from build123d import *

# Parameters (mm, degrees)
F0_W     = 60
F0_H     = 60
F0_R     = 2.2
F0_R_2   = 29
F1_DEPTH = 25
F3_DEPTH = 3


with BuildPart() as f1:
    # F0 (on Top) → F1 (new body)
    with BuildSketch(Plane.XY):
        Rectangle(F0_W, F0_H)
        with Locations((-25, -25)):
            Circle(F0_R, mode=Mode.SUBTRACT)
        with Locations((25, -25)):
            Circle(F0_R, mode=Mode.SUBTRACT)
        with Locations((-25, 25)):
            Circle(F0_R, mode=Mode.SUBTRACT)
        Circle(F0_R_2, mode=Mode.SUBTRACT)
        with Locations((25, 25)):
            Circle(F0_R, mode=Mode.SUBTRACT)
    extrude(amount=F1_DEPTH)

    # F2 (on face) → F3 (join)
    with BuildSketch(Plane.XY.offset(25)):
        with BuildLine():
            Line((-10, 27.221315), (-10, 0))
            ThreePointArc((-10, 0), (-9.293222, -3.692698), (-7.272797, -6.863412))
            Line((-7.272797, -6.863412), (-28.176117, -6.863412))
            ThreePointArc((-28.176117, -6.863412), (-27.743079, -8.445211), (-27.221315, -10))
            Line((-27.221315, -10), (0, -10))
            ThreePointArc((0, -10), (3.692698, -9.293222), (6.863412, -7.272797))
            Line((6.863412, -7.272797), (6.863412, -28.176117))
            ThreePointArc((6.863412, -28.176117), (8.445211, -27.743079), (10, -27.221315))
            Line((10, -27.221315), (10, 0))
            ThreePointArc((10, 0), (9.293222, 3.692698), (7.272797, 6.863412))
            Line((7.272797, 6.863412), (28.176117, 6.863412))
            ThreePointArc((28.176117, 6.863412), (27.743079, 8.445211), (27.221315, 10))
            Line((27.221315, 10), (0, 10))
            ThreePointArc((0, 10), (-3.692698, 9.293222), (-6.863412, 7.272797))
            Line((-6.863412, 7.272797), (-6.863412, 28.176117))
            ThreePointArc((-6.863412, 28.176117), (-8.445211, 27.743079), (-10, 27.221315))
        make_face()
    extrude(amount=-F3_DEPTH)


solid = f1.part
The listing builds one solid part. Answer for the finished solid, in the listing's coordinates (mm). A direction names the side the tool comes from. Coordinates: 2 decimals unless noted, no trailing zeros. Loops run counter-clockwise (first coordinate to the right, second up) from the corner with the lowest first, then second, coordinate; pieces in that order, holes last. Notation, with made-up numbers: (-5, 25.5) -> (25, 25.5) arc R23 cw to (25, 63.5) -> close; hole circle Ø4 at (43.25, 34). An arc over 180 degrees is marked (long way). Answer in a Markdown table with one row per item. Add a question column.
1. The part is cut by section D-D, the plane y = -2. Write down the section's boundary in (x, z), then the cut area to 3 significant figures.
2. The part is cut by section C-C, the plane x = -3.5. Write down the section's boundary in (y, z).
3. Consider line 1 (Y direction, x = -24, z = 23.25); line 2 (X direction, y = 24, z = 19); line 3 (Y direction, x = 1, z = 18.75). Determine where each line is inside the solid, lowest interval first. Write a range as [from, to].
4. Determine the mould class of faces 4 (the cylindrical face through (-9.313, -3.643, 23.521)), 5 (the flat face through (30, 0, 12)), 6 (the flat face through (-25, 16, 0)) for opening direction X: +X half, -X half, draft (parallel to the pull), parting line (faces both ways), or undercut.
5. Flat-ended cylindrical pins translate along their axes: P1, Ø17, axis at x = 11.5, y = -14, coming from the -Z side; P2, Ø3.5, axis at x = -25, y = -25, coming from the +Z side. Find the tip coordinate at first contact, or state that the pin passes through.
6. The part is cut by section A-A, the plane z = 3.5. Write down the section's boundary in (x, y).
7. For faces 1 (the flat face through (-14, -10, 24)), 2 (the flat face through (0, 0, 25)), 3 (the flat face through (0, 0, 22)), determine the directions among +Z, -Z, +X, -X, +Y, -Y from which every point of the face is accessible in a straight line to the end or side of a thin tool.
8. The part is cut by section B-B, the plane y = -25. Write down the section's boundary in (x, z).
Answer below:
| question | item | result |
|---|---|---|
| 1 | outline | (-30, 0) -> (-28.93, 0) -> (-28.93, 25) -> (-30, 25) -> close; (-9.8, 22) -> (10, 22) -> (10, 25) -> (-9.8, 25) -> close; (28.93, 0) -> (30, 0) -> (30, 25) -> (28.93, 25) -> close |
| 1 | area | 113 mm2 |
| 2 | outline | (-30, 0) -> (-28.79, 0) -> (-28.79, 25) -> (-30, 25) -> close; (-10, 22) -> (9.37, 22) -> (9.37, 25) -> (-10, 25) -> close; (28.79, 0) -> (30, 0) -> (30, 25) -> (28.79, 25) -> close |
| 3 | line 1 | [-30, -26.96], [-23.04, -16.28], [-10, -6.86], [16.28, 23.04], [26.96, 30] |
| 3 | line 2 | [-30, -26.96], [-23.04, -16.28], [16.28, 23.04], [26.96, 30] |
| 3 | line 3 | [-30, -28.98], [28.98, 30] |
| 4 | face 4 | undercut |
| 4 | face 5 | +X half |
| 4 | face 6 | draft |
| 5 | P1 | z = 22 |
| 5 | P2 | through |
| 6 | outline | (-30, -30) -> (30, -30) -> (30, 30) -> (-30, 30) -> close; hole circle Ø58 at (0, 0); hole circle Ø4.4 at (-25, -25); hole circle Ø4.4 at (-25, 25); hole circle Ø4.4 at (25, -25); hole circle Ø4.4 at (25, 25) |
| 7 | face 1 | +Z, -Z |
| 7 | face 2 | +Z, +X, -X, +Y, -Y |
| 7 | face 3 | -Z |
| 8 | outline | (-30, 0) -> (-27.2, 0) -> (-27.2, 25) -> (-30, 25) -> close; (-22.8, 0) -> (-14.7, 0) -> (-14.7, 25) -> (-22.8, 25) -> close; (6.86, 22) -> (10, 22) -> (10, 25) -> (6.86, 25) -> close; (14.7, 0) -> (22.8, 0) -> (22.8, 25) -> (14.7, 25) -> close; (27.2, 0) -> (30, 0) -> (30, 25) -> (27.2, 25) -> close |
